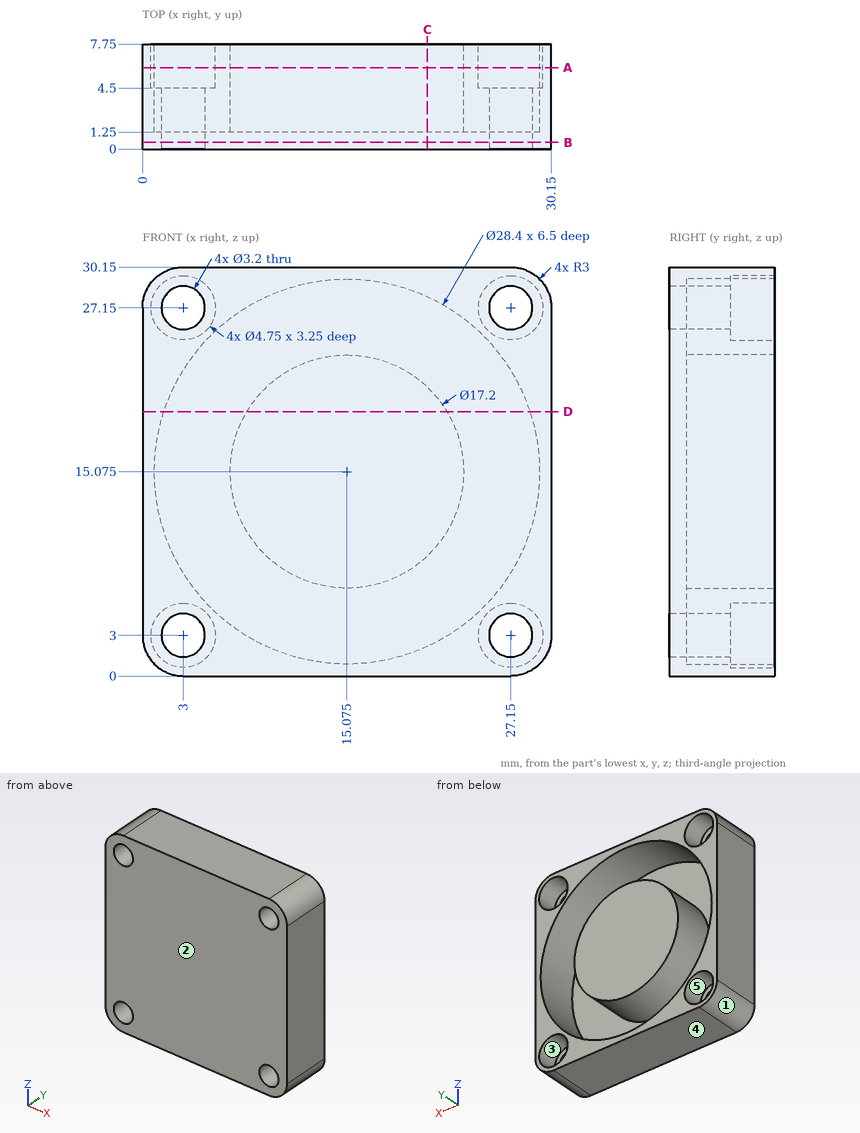
Part print with two shaded views. Sizes in mm from the minimum x, y, z corner. A direction names the side the tool comes from. Coordinates: 2 decimals unless noted, no trailing zeros. Write each loop counter-clockwise with the first axis right and the second up, starting at its lowest first coordinate (ties: lowest second). Pieces come first, ordered by that corner, then holes.
1. Band-saw the part on A-A, the plane y = 6. Give the cut face in (x, z) (3 decimals), and give its area (3 significant figures).
Answer block:
outline: (0, 3) arc R3 ccw to (3, 0) - (27.15, 0) arc R3 ccw to (30.15, 3) - (30.15, 27.15) arc R3 ccw to (27.15, 30.15) - (3, 30.15) arc R3 ccw to (0, 27.15) - close; circle Ø17.2 at (15.075, 15.075); hole circle Ø4.75 at (3, 3); hole circle Ø4.75 at (3, 27.15); hole circle Ø28.4 at (15.075, 15.075); hole circle Ø4.75 at (27.15, 3); hole circle Ø4.75 at (27.15, 27.15)
area: 429 mm2
2. Band-saw the part on D-D, the plane z = 19.5. Give the cut face in (x, y).
Answer block:
outline: (0, 0) - (30.15, 0) - (30.15, 7.75) - (28.57, 7.75) - (28.57, 1.25) - (22.45, 1.25) - (22.45, 7.75) - (7.7, 7.75) - (7.7, 1.25) - (1.58, 1.25) - (1.58, 7.75) - (0, 7.75) - close
3. Drill centre lines: probe 1 along X at (y, z) = (2, 15); probe 2 along X at (y, z) = (1.5, 11); probe 3 along X at (y, z) = (2.05, 27.15). Where is each one in solid material? Low to high.
Answer block:
probe 1: x = 0 to 0.88, 6.48 to 23.67, 29.27 to 30.15
probe 2: x = 0 to 1.47, 7.5 to 22.65, 28.68 to 30.15
probe 3: x = 0 to 1.4, 4.6 to 7.6, 22.55 to 25.55, 28.75 to 30.15
4. 3-axis set-ups, long thin cutter, end or side, ignore diameter. For the marked faces 4 and 5: which of +Z, -Z, +X, -X, +Y, -Y reach the whole face in a straight line?
Answer block:
face 4: -Z, +X, -X, +Y, -Y
face 5: +Y
5. Band-saw the part on B-B, the plane y = 0.5. Give the cut face in (x, z), and give its area (3 significant figures).
Answer block:
outline: (0, 3) arc R3 ccw to (3, 0) - (27.15, 0) arc R3 ccw to (30.15, 3) - (30.15, 27.15) arc R3 ccw to (27.15, 30.15) - (3, 30.15) arc R3 ccw to (0, 27.15) - close; hole circle Ø3.2 at (3, 3); hole circle Ø3.2 at (3, 27.15); hole circle Ø3.2 at (27.15, 3); hole circle Ø3.2 at (27.15, 27.15)
area: 869 mm2
6. Pull direction Z, two halves, no side cores. Call the marked faces 1, 2 and 3: released by +Z, released by -Z, zero draft, split by the parting line, or undercut.
Answer block:
face 1: released by -Z
face 2: zero draft
face 3: undercut
7. Drop flat-ended pins along their axis: pin 1 (3 mm diameter, centred on x = 27.15, z = 3, fed in from -Y); pin 2 (1.4 mm diameter, centred on x = 26.5, z = 4, fed in from +Y). Give the stop position or say it passes through.
Answer block:
pin 1: passes through
pin 2: stops at y = 4.5
8. Band-saw the part on C-C, the plane x = 21. Give the cut face in (y, z).
Answer block:
outline: (0, 0) - (7.75, 0) - (7.75, 2.17) - (1.25, 2.17) - (1.25, 8.84) - (7.75, 8.84) - (7.75, 21.31) - (1.25, 21.31) - (1.25, 27.98) - (7.75, 27.98) - (7.75, 30.15) - (0, 30.15) - close
